The figure shows three views and two pictorial views of one solid part (mm, origin at its lowest corner). Answer the questions. A direction names the side the tool comes from. Round coordinates to 2 decimals unless told otherwise and drop trailing zeros. Write each loop counter-clockwise with the first axis right and the second up, starting at its lowest first coordinate (ties: lowest second). Pieces come first, ordered by that corner, then holes.
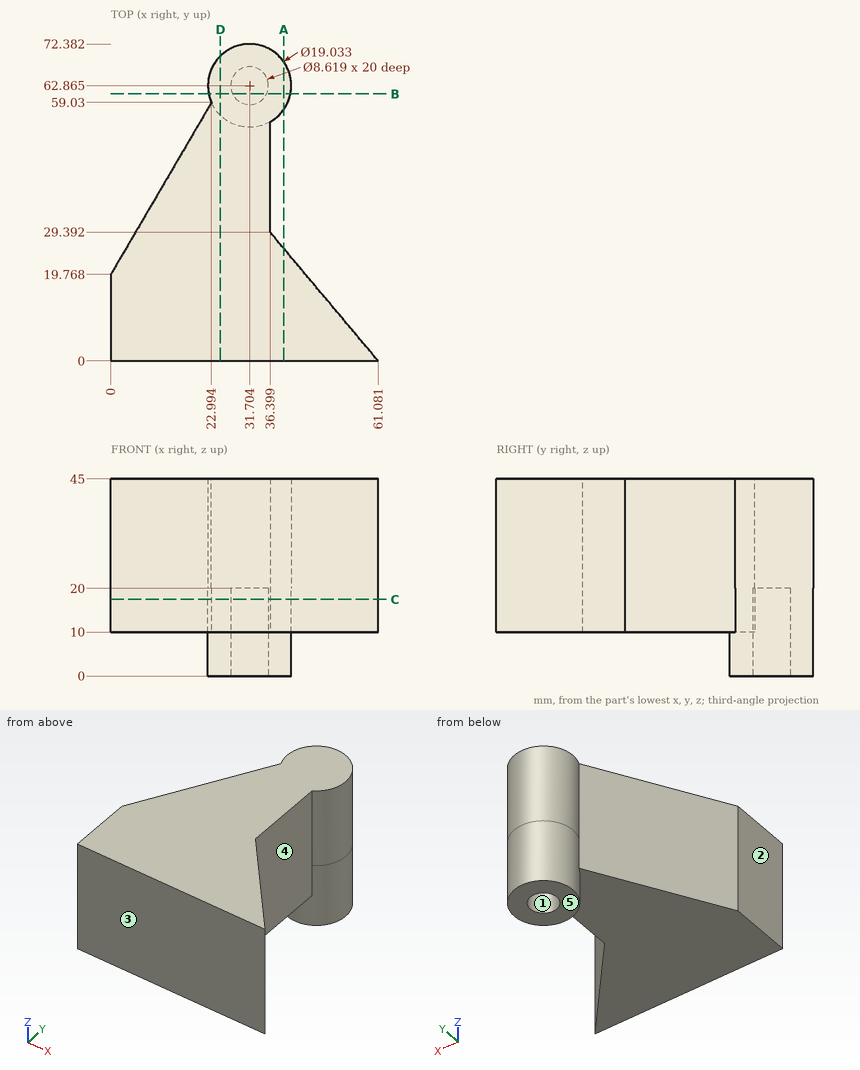
Q1. Section A-A (x = 39.5) is taken. Determine the outline of the cut face in (y, z), then the cut area to 3 significant figures.
Verdict:
outline: (0, 10) - (25.7, 10) - (25.7, 45) - (0, 45) - close; (57.41, 0) - (68.32, 0) - (68.32, 45) - (57.41, 45) - close
area: 1,390 mm2
Q2. Section B-B (y = 61) is taken. Determine the outline of the cut face in (x, z).
Verdict:
outline: (22.37, 0) - (27.82, 0) - (27.82, 20) - (35.59, 20) - (35.59, 0) - (41.04, 0) - (41.04, 45) - (22.37, 45) - close
Q3. Section D-D (x = 25) is taken. Determine the outline of the cut face in (y, z).
Verdict:
outline: (0, 10) - (56.11, 10) - (56.11, 0) - (69.62, 0) - (69.62, 45) - (0, 45) - close
Q4. Straight lines are drawn through the part: probe 1 along Y at (x, z) = (31.5, 8.5); probe 2 along Y at (x, z) = (39, 37) (1 decimal); probe 3 along Z at (x, y) = (35, 45.5). For each, find the intervals that lie inside material, in ascending order.
Verdict:
probe 1: y = 53.35 to 58.56, 67.17 to 72.38
probe 2: y = 0 to 26.3, 56.8 to 69
probe 3: z = 10 to 45
Q5. Flat-ended cylindrical pins translate along their axes: pin 1 Ø10 at (x, z) = (27, 39) entering from -Y; pin 2 Ø3 at (x, z) = (53, 22) entering from +Y; pin 3 Ø20 at (y, z) = (47.5, 25) entering from +X (1 decimal); pin 4 Ø12 at (y, z) = (42.5, 30) entering from +X. Find the tip coordinate at first contact, or state that the pin passes through.
Verdict:
pin 1: stops at y = 0
pin 2: stops at y = 11.41
pin 3: stops at x = 39.6
pin 4: stops at x = 36.4
Q6. Section C-C (z = 17.5) is taken. Determine the outline of the cut face in (x, y) (1 decimal), then the cut area to 3 significant figures.
Verdict:
outline: (0, 0) - (61.1, 0) - (36.4, 29.4) - (36.4, 54.6) arc R9.5 ccw (long way) to (23, 59) - (0, 19.8) - close; hole circle Ø8.6 at (31.7, 62.9)
area: 2,230 mm2
Q7. Determine the mould class of the marked faces 3, 4 and 5 for opening direction Y: pulls with the +Y half, pulls with the -Y half, needs draft (parallel to the pull), parting line crosses it, or undercut.
Verdict:
face 3: pulls with the -Y half
face 4: undercut
face 5: needs draft
Q8. Which of the six approach directions +Z, -Z, +X, -X, +Y, -Y give full straight-line access (tool end or side, diameter ignored) to the marked faces 1 and 2?
Verdict:
face 1: -Z
face 2: +Z, -Z, -X, +Y, -Y
